from build123d import *

# Parameters (mm, degrees)
BOSS_EXTRUDE1_DEPTH = 50
SKETCH3_R           = 4
CUT_EXTRUDE1_DEPTH  = 84.815273071
SKETCH2_R           = 4
CUT_EXTRUDE2_DEPTH  = 200


with BuildPart() as part:
    # Sketch1 → Boss-Extrude1 (new, symmetric)
    with BuildSketch(Plane.XY):
        Polygon((0, 50), (5, 50), (5, 5), (50, 5), (50, 0), (0, 0), align=None)
    extrude(amount=BOSS_EXTRUDE1_DEPTH, both=True)

    # Sketch3 → Cut-Extrude1 (cut, through all)
    with BuildSketch(Plane(origin=(0, 5, 0), x_dir=(1, 0, 0), z_dir=(0, 1, 0))):
        with Locations(Location((35, 25, 0), (0, 0, 180))):
            Circle(SKETCH3_R)
        with Locations(Location((35, -25, 0), (0, 0, 180))):
            Circle(SKETCH3_R)
    extrude(amount=-CUT_EXTRUDE1_DEPTH, mode=Mode.SUBTRACT)

    # Sketch2 → Cut-Extrude2 (cut)
    with BuildSketch(Plane(origin=(5, 0, 0), x_dir=(0, 0, -1), z_dir=(1, 0, 0))):
        with Locations(Location((-25, 35, 0), (0, 0, 90))):
            Circle(SKETCH2_R)
        with Locations(Location((25, 35, 0), (0, 0, 90))):
            Circle(SKETCH2_R)
    extrude(amount=-CUT_EXTRUDE2_DEPTH, mode=Mode.SUBTRACT)


solid = part.part
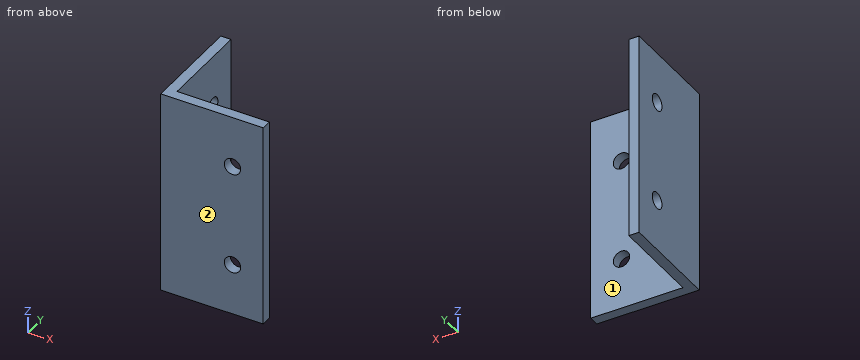
Input: part model. Units: mm. Frame: model coordinates. Face numbers are marked on the shaded views. A direction names the side the tool comes from. Give positions to 0.01 mm unless a question says otherwise; leave off trailing zeros. Order: outer loops, then holes, each group sorted by start corner. A loop starts at its lowest first (then second) coordinate and runs counter-clockwise, first axis right, second up. Notation, with made-up numbers: M -28.5,85.5 L -23.5,85.5 A22 ccw -23.5,119.5 Z; hole C -1,-25 d1. An arc over 180 degrees is marked long. Answer as a JSON object with one key per item and string values.
1. Cut plane A-A, the plane x = 35. Output: boundary loops of the cut face in (y, z), and give its area (3 significant figures).
Result sheet:
{"outline": "M 0,-50 L 5,-50 L 5,-29 L 0,-29 Z; M 0,-21 L 5,-21 L 5,21 L 0,21 Z; M 0,29 L 5,29 L 5,50 L 0,50 Z", "area": "420 mm²"}
2. Ray query, line 1 (Z direction, x = 3, y = 35); line 2 (X direction, y = 15.5, z = -13). Return the intervals inside material, ascending. Write a range as [from, to].
Result sheet:
{"line 1": "[-50, -29], [-21, 21], [29, 50]", "line 2": "[0, 5]"}
3. Cut plane B-B, the plane z = 25. Output: boundary loops of the cut face in (x, y).
Result sheet:
{"outline": "M 0,0 L 31,0 L 31,5 L 5,5 L 5,31 L 0,31 Z; M 0,39 L 5,39 L 5,50 L 0,50 Z; M 39,0 L 50,0 L 50,5 L 39,5 Z"}
4. Reachability of the marked faces 1 and 2 from +Z, -Z, +X, -X, +Y, -Y: full face, straight path, thin tool, end or side. Return the list, or none.
Result sheet:
{"face 1": "+Z, -Z, +X, +Y", "face 2": "+Z, -Z, +X, -X, -Y"}
5. Cut plane D-D, the plane z = 35. Output: boundary loops of the cut face in (x, y).
Result sheet:
{"outline": "M 0,0 L 50,0 L 50,5 L 5,5 L 5,50 L 0,50 Z"}
6. First-contact query: P1, Ø13, axis at y = 35, z = -25, coming from the +X side; P2, Ø4, axis at x = 36, z = 22.5, coming from the +Y side. Flat tips, straight axial feed; report the tip coordinate or a pass-through.
Result sheet:
{"P1": "x = 5", "P2": "y = 5"}
